Geometry check sheet. Reference: the model listing, model coordinates, mm. Round coordinates to 2 decimals unless told otherwise and drop trailing zeros. Write each loop counter-clockwise with the first axis right and the second up, starting at its lowest first coordinate (ties: lowest second). Pieces come first, ordered by that corner, then holes. Notation, with made-up numbers: M 22,7 L 48,7 A32 ccw 48,43 Z; hole C 83,-38.5 d10. An arc over 180 degrees is marked long. Answer in a Markdown table with one row per item. Add a question column.
from build123d import *

# Parameters (mm, degrees)
BOSS_EXTRUDE1_DEPTH = 3
CUT_EXTRUDE1_REACH  = 242.652
SKETCH2_R           = 2.5
CUT_EXTRUDE2_REACH  = 242.652
CUT_EXTRUDE3_REACH  = 242.652


with BuildPart() as part:
    # Sketch1 → Boss-Extrude1 (new body)
    with BuildSketch(Plane(origin=(0, 0, 0), x_dir=(0, 0, -1), z_dir=(1, 0, 0))):
        with BuildLine():
            Line((-12.188515962, 194.5), (106.683660563, 194.5))
            ThreePointArc((106.683660563, 194.5), (131.432397904, 184.248737342), (141.683660563, 159.5))
            Line((141.683660563, 159.5), (141.683660563, 20))
            ThreePointArc((141.683660563, 20), (131.432397904, -4.748737342), (106.683660563, -15))
            Line((106.683660563, -15), (-106.683660563, -15))
            ThreePointArc((-106.683660563, -15), (-128.230433314, -2.678193247), (-128.537592466, 22.141073279))
            Line((-128.537592466, 22.141073279), (-42.784020626, 176.497502591))
            ThreePointArc((-42.784020626, 176.497502591), (-29.937986507, 189.665481852), (-12.188515962, 194.5))
        make_face()
    extrude(amount=BOSS_EXTRUDE1_DEPTH)

    # Sketch2 → Cut-Extrude1 (cut, up to next)
    with BuildSketch(Plane(origin=(3, 0, 0), x_dir=(0, 0, -1), z_dir=(1, 0, 0)), mode=Mode.PRIVATE) as cut_extrude1_sk1:
        with Locations((81.683660563, 184.5)):
            Circle(SKETCH2_R)
    cut_extrude1_tool1 = extrude(cut_extrude1_sk1.sketch, amount=-CUT_EXTRUDE1_REACH, mode=Mode.PRIVATE) & part.part
    # Sketch2 → Cut-Extrude1 (cut, up to next)
    with BuildSketch(Plane(origin=(3, 0, 0), x_dir=(0, 0, -1), z_dir=(1, 0, 0)), mode=Mode.PRIVATE) as cut_extrude1_sk2:
        with Locations((12.811484038, 184.5)):
            Circle(SKETCH2_R)
    cut_extrude1_tool2 = extrude(cut_extrude1_sk2.sketch, amount=-CUT_EXTRUDE1_REACH, mode=Mode.PRIVATE) & part.part
    # Sketch2 → Cut-Extrude1 (cut, up to next)
    with BuildSketch(Plane(origin=(3, 0, 0), x_dir=(0, 0, -1), z_dir=(1, 0, 0)), mode=Mode.PRIVATE) as cut_extrude1_sk3:
        with Locations((131.683660563, 134.49995686)):
            Circle(SKETCH2_R)
    cut_extrude1_tool3 = extrude(cut_extrude1_sk3.sketch, amount=-CUT_EXTRUDE1_REACH, mode=Mode.PRIVATE) & part.part
    # Sketch2 → Cut-Extrude1 (cut, up to next)
    with BuildSketch(Plane(origin=(3, 0, 0), x_dir=(0, 0, -1), z_dir=(1, 0, 0)), mode=Mode.PRIVATE) as cut_extrude1_sk4:
        with Locations((131.683660563, 89.75)):
            Circle(SKETCH2_R)
    cut_extrude1_tool4 = extrude(cut_extrude1_sk4.sketch, amount=-CUT_EXTRUDE1_REACH, mode=Mode.PRIVATE) & part.part
    # Sketch2 → Cut-Extrude1 (cut, up to next)
    with BuildSketch(Plane(origin=(3, 0, 0), x_dir=(0, 0, -1), z_dir=(1, 0, 0)), mode=Mode.PRIVATE) as cut_extrude1_sk5:
        with Locations((131.683660563, 44.999939605)):
            Circle(SKETCH2_R)
    cut_extrude1_tool5 = extrude(cut_extrude1_sk5.sketch, amount=-CUT_EXTRUDE1_REACH, mode=Mode.PRIVATE) & part.part
    # Sketch2 → Cut-Extrude1 (cut, up to next)
    with BuildSketch(Plane(origin=(3, 0, 0), x_dir=(0, 0, -1), z_dir=(1, 0, 0)), mode=Mode.PRIVATE) as cut_extrude1_sk6:
        with Locations((71.683660563, -5)):
            Circle(SKETCH2_R)
    cut_extrude1_tool6 = extrude(cut_extrude1_sk6.sketch, amount=-CUT_EXTRUDE1_REACH, mode=Mode.PRIVATE) & part.part
    # Sketch2 → Cut-Extrude1 (cut, up to next)
    with BuildSketch(Plane(origin=(3, 0, 0), x_dir=(0, 0, -1), z_dir=(1, 0, 0)), mode=Mode.PRIVATE) as cut_extrude1_sk7:
        with Locations((0, -5)):
            Circle(SKETCH2_R)
    cut_extrude1_tool7 = extrude(cut_extrude1_sk7.sketch, amount=-CUT_EXTRUDE1_REACH, mode=Mode.PRIVATE) & part.part
    # Sketch2 → Cut-Extrude1 (cut, up to next)
    with BuildSketch(Plane(origin=(3, 0, 0), x_dir=(0, 0, -1), z_dir=(1, 0, 0)), mode=Mode.PRIVATE) as cut_extrude1_sk8:
        with Locations((-71.683660563, -5)):
            Circle(SKETCH2_R)
    cut_extrude1_tool8 = extrude(cut_extrude1_sk8.sketch, amount=-CUT_EXTRUDE1_REACH, mode=Mode.PRIVATE) & part.part
    # Sketch2 → Cut-Extrude1 (cut, up to next)
    with BuildSketch(Plane(origin=(3, 0, 0), x_dir=(0, 0, -1), z_dir=(1, 0, 0)), mode=Mode.PRIVATE) as cut_extrude1_sk9:
        with Locations((-100.370302458, 52.250935013)):
            Circle(SKETCH2_R)
    cut_extrude1_tool9 = extrude(cut_extrude1_sk9.sketch, amount=-CUT_EXTRUDE1_REACH, mode=Mode.PRIVATE) & part.part
    # Sketch2 → Cut-Extrude1 (cut, up to next)
    with BuildSketch(Plane(origin=(3, 0, 0), x_dir=(0, 0, -1), z_dir=(1, 0, 0)), mode=Mode.PRIVATE) as cut_extrude1_sk10:
        with Locations((-76.919233785, 94.462858624)):
            Circle(SKETCH2_R)
    cut_extrude1_tool10 = extrude(cut_extrude1_sk10.sketch, amount=-CUT_EXTRUDE1_REACH, mode=Mode.PRIVATE) & part.part
    # Sketch2 → Cut-Extrude1 (cut, up to next)
    with BuildSketch(Plane(origin=(3, 0, 0), x_dir=(0, 0, -1), z_dir=(1, 0, 0)), mode=Mode.PRIVATE) as cut_extrude1_sk11:
        with Locations((-53.468165112, 136.674782235)):
            Circle(SKETCH2_R)
    cut_extrude1_tool11 = extrude(cut_extrude1_sk11.sketch, amount=-CUT_EXTRUDE1_REACH, mode=Mode.PRIVATE) & part.part
    add(cut_extrude1_tool1.solids().sort_by_distance((3, 184.5, -81.683661))[0], mode=Mode.SUBTRACT)
    add(cut_extrude1_tool2.solids().sort_by_distance((3, 184.5, -12.811484))[0], mode=Mode.SUBTRACT)
    add(cut_extrude1_tool3.solids().sort_by_distance((3, 134.499957, -131.683661))[0], mode=Mode.SUBTRACT)
    add(cut_extrude1_tool4.solids().sort_by_distance((3, 89.75, -131.683661))[0], mode=Mode.SUBTRACT)
    add(cut_extrude1_tool5.solids().sort_by_distance((3, 44.99994, -131.683661))[0], mode=Mode.SUBTRACT)
    add(cut_extrude1_tool6.solids().sort_by_distance((3, -5, -71.683661))[0], mode=Mode.SUBTRACT)
    add(cut_extrude1_tool7.solids().sort_by_distance((3, -5, 0))[0], mode=Mode.SUBTRACT)
    add(cut_extrude1_tool8.solids().sort_by_distance((3, -5, 71.683661))[0], mode=Mode.SUBTRACT)
    add(cut_extrude1_tool9.solids().sort_by_distance((3, 52.250935, 100.370302))[0], mode=Mode.SUBTRACT)
    add(cut_extrude1_tool10.solids().sort_by_distance((3, 94.462859, 76.919234))[0], mode=Mode.SUBTRACT)
    add(cut_extrude1_tool11.solids().sort_by_distance((3, 136.674782, 53.468165))[0], mode=Mode.SUBTRACT)

    # Sketch4 → Cut-Extrude2 (cut, up to next)
    with BuildSketch(Plane(origin=(3, 0, 0), x_dir=(0, 0, -1), z_dir=(1, 0, 0)), mode=Mode.PRIVATE) as cut_extrude2_sk1:
        with BuildLine():
            Line((141.683660563, 144.5), (126.683660563, 144.5))
            Line((126.683660563, 144.5), (126.683660563, 159.5))
            ThreePointArc((126.683660563, 159.5), (120.825796187, 173.642135624), (106.683660563, 179.5))
            Line((106.683660563, 179.5), (91.683660563, 179.5))
            Line((91.683660563, 179.5), (91.683660563, 194.5))
            Line((91.683660563, 194.5), (141.683660563, 194.5))
            Line((141.683660563, 194.5), (141.683660563, 144.5))
        make_face()
    cut_extrude2_tool1 = extrude(cut_extrude2_sk1.sketch, amount=-CUT_EXTRUDE2_REACH, mode=Mode.PRIVATE) & part.part
    add(cut_extrude2_tool1.solids().sort_by_distance((3, 176.600336, -123.783996))[0], mode=Mode.SUBTRACT)

    # Sketch5 → Cut-Extrude3 (cut, up to next)
    with BuildSketch(Plane(origin=(3, 0, 0), x_dir=(0, 0, -1), z_dir=(1, 0, 0)), mode=Mode.PRIVATE) as cut_extrude3_sk1:
        with BuildLine():
            Line((106.683660563, 179.5), (126.683660563, 159.5))
            ThreePointArc((126.683660563, 159.5), (120.825796187, 173.642135624), (106.683660563, 179.5))
        make_face()
    cut_extrude3_tool1 = extrude(cut_extrude3_sk1.sketch, amount=-CUT_EXTRUDE3_REACH, mode=Mode.PRIVATE) & part.part
    add(cut_extrude3_tool1.solids().sort_by_distance((3, 171.179589, -118.36325))[0], mode=Mode.SUBTRACT)


solid = part.part
Item 1: Gauge pin test, flat ends, axial feed: pin 1 Ø0.9 at (x, y) = (2, 186) entering from -Z; pin 2 Ø1.5 at (x, y) = (0.5, 8.5) entering from -Z. Record the tip position at first contact, or that the pin passes through.
Item 2: Scan lines: probe 1 along Y at (x, z) = (2.2, 0); probe 2 along Y at (x, z) = (1.6, -2); probe 3 along Z at (x, y) = (2.4, 34). Record each from-to range of solid material in increasing order. Write a range as from..to.
Item 3: Section check B-B, the plane y = 167. Record the boundary of the cut face in (x, z), and give its area (3 significant figures).
Item 4: Section check C-C, the plane z = 28. Record the boundary of the cut face in (x, y).
Item 5: Section check A-A, the plane x = 1.9. Give the number of separate pieces and of enclosed holes in the cut face, and give its area (3 significant figures).
Result sheet:
| question | item | result |
|---|---|---|
| 1 | pin 1 | stops at z = -91.68 |
| 1 | pin 2 | stops at z = -139.99 |
| 2 | probe 1 | y = -15..-7.5, -2.5..194.5 |
| 2 | probe 2 | y = -15..-6.5, -3.5..194.5 |
| 2 | probe 3 | z = -141.68..121.95 |
| 3 | outline | M 0,-119.18 L 3,-119.18 L 3,48.06 L 0,48.06 Z |
| 3 | area | 502 mm^2 |
| 4 | outline | M 0,-15 L 3,-15 L 3,190.72 L 0,190.72 Z |
| 5 | separate pieces | 1 |
| 5 | enclosed holes | 11 |
| 5 | area | 46,300 mm^2 |
